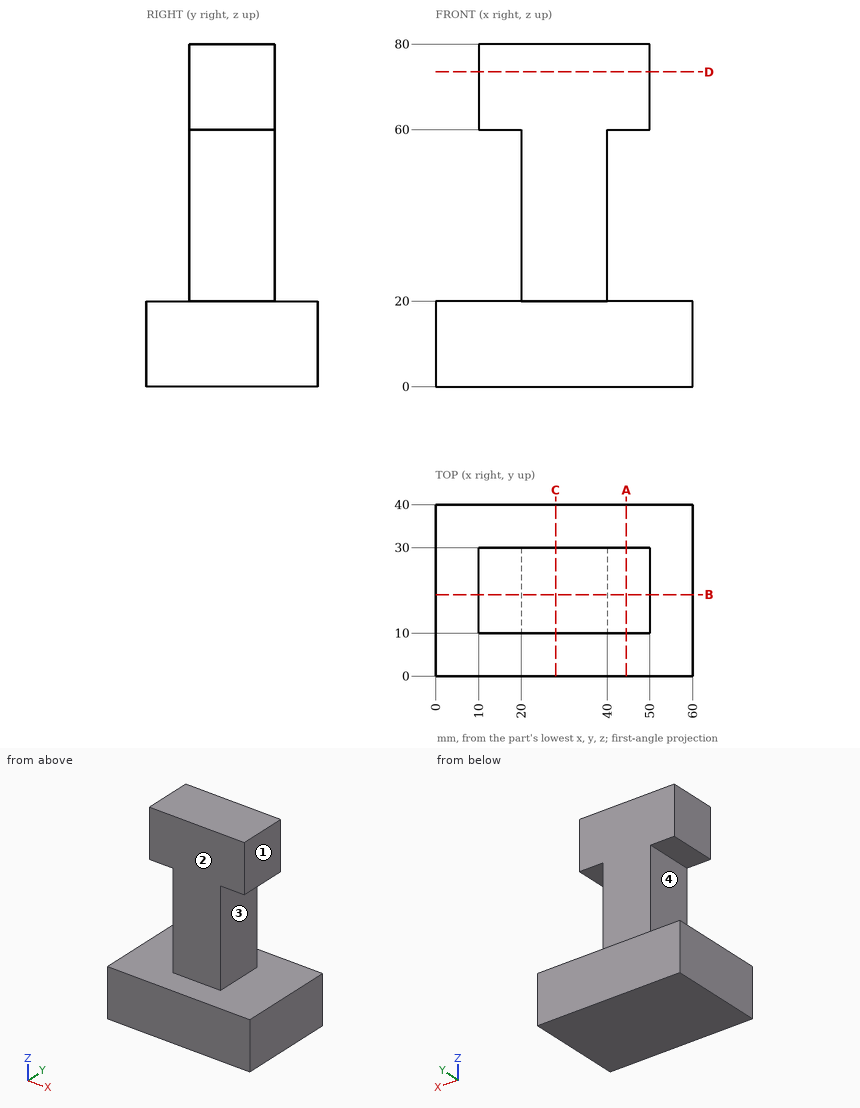
Design review of the part shown in the three views and the two pictorial views. Dimensions are in mm from the part's minimum x, y and z. A direction names the side the tool comes from. Give positions to 0.01 mm unless a question says otherwise; leave off trailing zeros. Loops run counter-clockwise (first coordinate to the right, second up) from the corner with the lowest first, then second, coordinate; pieces in that order, holes last. Notation, with made-up numbers: M 56,41.25 L 92,41.25 A35 cw 92,78.25 Z; hole C 69.25,79 d11. An arc over 180 degrees is marked long. Answer as a JSON object with one key per item and string values. Group by question number.
Q1. For probe 1 along Z at (x, y) = (17.5, 26); probe 2 along Z at (x, y) = (55.5, 19); probe 3 along Y at (x, z) = (30.5, 62), list the stretches that pass through material, from the lowest coordinate up. Write a range as [from, to].
Q2. Add section B-B on y = 19. Give the boundary of the cut face in (x, z).
Q3. Tool access review of the marked faces 1, 2, 3 and 4: name each direction out of +Z, -Z, +X, -X, +Y, -Y from which nothing blocks a thin tool from reaching the whole face with its end or side.
Q4. Add section A-A on x = 44.5. Give the boundary of the cut face in (y, z).
Q5. Insertion check: P1, Ø2, axis at x = 38, z = 33.5, coming from the -Y side; P2, Ø12, axis at x = 36.5, z = 55, coming from the +Y side; P3, Ø8, axis at y = 21.5, z = 68, coming from the +X side. Each pin has a flat end and moves straight along its axis. Give the tip position at first contact, or say it passes through.
Q6. Add section C-C on x = 28. Give the boundary of the cut face in (y, z), and give its area (3 significant figures).
Q7. Add section D-D on z = 73.5. Give the boundary of the cut face in (x, y), and give its area (3 significant figures).
Checked values:
{
 "1": {"probe 1": "[0, 20], [60, 80]", "probe 2": "[0, 20]", "probe 3": "[10, 30]"},
 "2": {"outline": "M 0,0 L 60,0 L 60,20 L 40,20 L 40,60 L 50,60 L 50,80 L 10,80 L 10,60 L 20,60 L 20,20 L 0,20 Z"},
 "3": {"face 1": "+Z, +X, +Y, -Y", "face 2": "+Z, +X, -X, -Y", "face 3": "+X, +Y, -Y", "face 4": "-X, +Y, -Y"},
 "4": {"outline": "M 0,0 L 40,0 L 40,20 L 0,20 Z; M 10,60 L 30,60 L 30,80 L 10,80 Z"},
 "5": {"P1": "y = 10", "P2": "y = 30", "P3": "x = 50"},
 "6": {"outline": "M 0,0 L 40,0 L 40,20 L 30,20 L 30,80 L 10,80 L 10,20 L 0,20 Z", "area": "2,000 mm²"},
 "7": {"outline": "M 10,10 L 50,10 L 50,30 L 10,30 Z", "area": "800 mm²"}
}
